```python
from build123d import *

# Parameters (mm, degrees)
SKETCH_1_R      = 3
SKETCH_1_R_2    = 1.75
EXTRUDE_1_DEPTH = 3
SKETCH_4_R      = 3
EXTRUDE_3_DEPTH = 10
EXTRUDE_5_REACH = 37.51


with BuildPart() as part:
    # 草图1 → 凸台-拉伸1 (new body)
    with BuildSketch(Plane(origin=(0, 0, 0), x_dir=(1, 0, 0), z_dir=(0, 1, 0))):
        with BuildLine():
            Line((-6.251193562, -12.539301448), (18.001154819, -4.761126855))
            ThreePointArc((18.001154819, -4.761126855), (21.333794073, -1.176473834), (20.009707694, 3.535533906))
            Line((20.009707694, 3.535533906), (3.535533906, 20.009707694))
            ThreePointArc((3.535533906, 20.009707694), (-1.176473834, 21.333794073), (-4.761126855, 18.001154819))
            Line((-4.761126855, 18.001154819), (-12.539301448, -6.251193562))
            ThreePointArc((-12.539301448, -6.251193562), (-11.313708499, -11.313708499), (-6.251193562, -12.539301448))
        make_face()
        with Locations(Location((0, 0, 0), (0, 0, 270))):
            Circle(SKETCH_1_R, mode=Mode.SUBTRACT)
        with Locations(Location((0, 16.474173788, 0), (0, 0, 270))):
            Circle(SKETCH_1_R_2, mode=Mode.SUBTRACT)
        with Locations(Location((16.474173788, 0, 0), (0, 0, 270))):
            Circle(SKETCH_1_R_2, mode=Mode.SUBTRACT)
        with Locations(Location((-7.778174593, -7.778174593, 0), (0, 0, 270))):
            Circle(SKETCH_1_R_2, mode=Mode.SUBTRACT)
    extrude(amount=EXTRUDE_1_DEPTH)

    # 草图4 → 凸台-拉伸3 (add)
    with BuildSketch(Plane(origin=(0, 3, 0), x_dir=(1, 0, 0), z_dir=(0, 1, 0))):
        with BuildLine():
            ThreePointArc((-1.03695933, 13.436395181), (-2.822849114, 13.143867789), (-3.641592762, 11.529980113))
            Line((-3.641592762, 11.529980113), (-3.641592762, 10.493))
            Line((-3.641592762, 10.493), (4.358407238, 10.493))
            Line((4.358407238, 10.493), (4.358407238, 5.293))
            Line((4.358407238, 5.293), (-3.641592762, 5.293))
            Line((-3.641592762, 5.293), (-3.641592762, -3.641592762))
            Line((-3.641592762, -3.641592762), (5.293, -3.641592762))
            Line((5.293, -3.641592762), (5.293, 4.358407238))
            Line((5.293, 4.358407238), (10.493, 4.358407238))
            Line((10.493, 4.358407238), (10.493, -3.641592762))
            Line((10.493, -3.641592762), (11.529980113, -3.641592762))
            ThreePointArc((11.529980113, -3.641592762), (13.143867789, -2.822849114), (13.436395181, -1.03695933))
            Line((13.436395181, -1.03695933), (10.264822306, 8.96304067))
            ThreePointArc((10.264822306, 8.96304067), (9.7726208, 9.7726208), (8.96304067, 10.264822306))
            Line((8.96304067, 10.264822306), (-1.03695933, 13.436395181))
        make_face()
        Circle(SKETCH_4_R, mode=Mode.SUBTRACT)
    extrude(amount=EXTRUDE_3_DEPTH)

    # 草图8 → 凸台-拉伸5 (add, up to next)
    with BuildSketch(Plane.XY.offset(3.641592762), mode=Mode.PRIVATE) as extrude_5_sk1:
        with BuildLine():
            ThreePointArc((10.493, 9.7), (7.893, 7.1), (5.293, 9.7))
            Line((5.293, 9.7), (5.293, 3))
            Line((5.293, 3), (10.493, 3))
            Line((10.493, 3), (10.493, 9.7))
        make_face()
    extrude_5_tool1 = extrude(extrude_5_sk1.sketch, amount=-EXTRUDE_5_REACH, mode=Mode.PRIVATE) - part.part
    extrude_5 = extrude_5_tool1.solids().sort_by_distance((7.893, 5.365131, 3.641593))[0]
    add(extrude_5)

    # 镜向7: 凸台-拉伸5 across plane
    add(extrude_5.mirror(Plane(origin=(0, 0, 0), x_dir=(-0.7071067811865476, 0, 0.7071067811865475), z_dir=(0.7071067811865475, 0, 0.7071067811865476))))


solid = part.part
```
Verification items for the finished model (mm, model axes). A direction names the side the tool comes from. Coordinates: 2 decimals unless noted, no trailing zeros. Order: outer loops, then holes, each group sorted by start corner. A loop starts at its lowest first (then second) coordinate and runs counter-clockwise, first axis right, second up. Notation, with made-up numbers: (40.5, -29) - (93.5, -29) arc R30 cw to (93.5, 2) - close; hole circle Ø4 at (-31.5, 77). An arc over 180 degrees is marked (long way). Return JSON: item names as keys, results as strings.
(1) Go/stop test with flat-tipped pins: pin 1 (3.5 mm diameter, centred on x = -1, y = 11.5, fed in from +Z); pin 2 (6 mm diameter, centred on x = 11.5, y = 3.5, fed in from -Z); pin 3 (3.5 mm diameter, centred on y = 12, z = 0, fed in from +X); pin 4 (4 mm diameter, centred on x = 0, z = -16.47, fed in from -Y). Record where each tip stops, or that it passes through.
Filled sheet:
{"pin 1": "stops at z = 3.64", "pin 2": "stops at z = -15", "pin 3": "stops at x = 13.53", "pin 4": "stops at y = 0"}
(2) Thickness scan on line 1 along X through (y, z) = (7.75, 0); line 2 along Z through (x, y) = (2.5, 8.75); line 3 along Y through (x, z) = (-1, 8). Record the ranges inside material, lowest first.
Filled sheet:
{"line 1": "x = -3.64 to -3, 3 to 6.17, 9.61 to 13.11", "line 2": "z = -12.31 to -10.31, -5.47 to -1.66, 1.66 to 3.64", "line 3": "y = 0 to 3"}
(3) Section check D-D, the plane y = 8.5. Record the cut outline in (x, z).
Filled sheet:
{"outline": "(-3.64, -11.53) arc R2 ccw to (-1.04, -13.44) - (8.96, -10.26) arc R2 ccw to (10.26, -8.96) - (13.44, 1.04) arc R2 ccw to (11.53, 3.64) - (10.2, 3.64) - (10.2, -4.36) - (5.59, -4.36) - (5.59, 3.64) - (-3.64, 3.64) - (-3.64, -5.59) - (4.36, -5.59) - (4.36, -10.2) - (-3.64, -10.2) - close; hole circle Ø6 at (0, 0)"}
(4) Section check A-A, the plane y = 12. Record the cut outline in (x, z), and give its area (3 significant figures).
Filled sheet:
{"outline": "(-3.64, -11.53) arc R2 ccw to (-1.04, -13.44) - (8.96, -10.26) arc R2 ccw to (10.26, -8.96) - (13.44, 1.04) arc R2 ccw to (11.53, 3.64) - (10.49, 3.64) - (10.49, -4.36) - (5.29, -4.36) - (5.29, 3.64) - (-3.64, 3.64) - (-3.64, -5.29) - (4.36, -5.29) - (4.36, -10.49) - (-3.64, -10.49) - close; hole circle Ø6 at (0, 0)", "area": "128 mm^2"}
(5) Mould release check, pull along Z, two halves, no side actions. Record for faces 1 (the cylindrical face through (0.3, 7.1, -7.95)), 2 (the flat face through (5, 13, -5)), 3 (the flat face through (5.705, 1.479, 8.705)): pulls with the +Z half, pulls with the -Z half, needs draft (parallel to the pull), parting line crosses it, or undercut.
Filled sheet:
{"face 1": "undercut", "face 2": "needs draft", "face 3": "pulls with the +Z half"}
(6) Access from +Z, -Z, +X, -X, +Y, -Y to the whole of each face (thin tool, end or side, straight path). Record for faces 4 (the cylindrical face through (9.782, 7.93, -9.763)), 5 (the cylindrical face through (-3, 8, -13)), 6 (the flat face through (5.293, 11, 0)).
Filled sheet:
{"face 4": "-Z, +X, +Y", "face 5": "-Z, +Y", "face 6": "+Z, +Y"}
(7) Section check C-C, the plane z = -6. Record the cut outline in (x, y), and give its area (3 significant figures).
Filled sheet:
{"outline": "(-8.61, 0) - (17.55, 0) - (17.55, 3) - (11.2, 3) - (11.2, 13) - (4.36, 13) - (4.36, 7.92) - (-3.64, 7.92) - (-3.64, 3) - (-8.61, 3) - close", "area": "186 mm^2"}
